Part print with two shaded views. Sizes in mm from the minimum x, y, z corner. Coordinates: 2 decimals unless noted, no trailing zeros. Write each loop counter-clockwise with the first axis right and the second up, starting at its lowest first coordinate (ties: lowest second). Pieces come first, ordered by that corner, then holes. Notation, with made-up numbers: M 80.25,19.5 L 101.25,19.5 A6 cw 101.25,23.5 Z; hole C 10,81.25 d7. An arc over 180 degrees is marked long. One line per question, with ' | ' between items. Start each with the question number.
(1) Cut at A-A (x = 18.5). Write the cut outline in (y, z), plus the area to 3 significant figures.
(2) Wall check: probe 1 along X at (y, z) = (2, 18.5); probe 2 along Z at (x, y) = (19, 1); probe 3 along Z at (x, y) = (13.5, 4). Give the ranges that are in metal, low to high.
(3) Cut at B-B (z = 18.5). Write the cut outline in (x, y), plus the area to 3 significant figures.
(4) Flat gauge pins, fed straight in: pin 1 Ø3 at (x, y) = (6, 5.5) entering from +Z; pin 2 Ø1.5 at (x, y) = (25.5, 1) entering from +Z; pin 3 Ø1.5 at (y, z) = (3, 29.5) entering from -X. Where does each tip first touch, or does it go through?
(5) Cut at C-C (y = 4). Write the cut outline in (x, z), plus the area to 3 significant figures.
(6) Two-plate mould, pull along Z, no slides. Class the marked faces 1, 2 and 3: +Z half, -Z half, draft (parallel to the pull), parting line (faces both ways), or undercut.
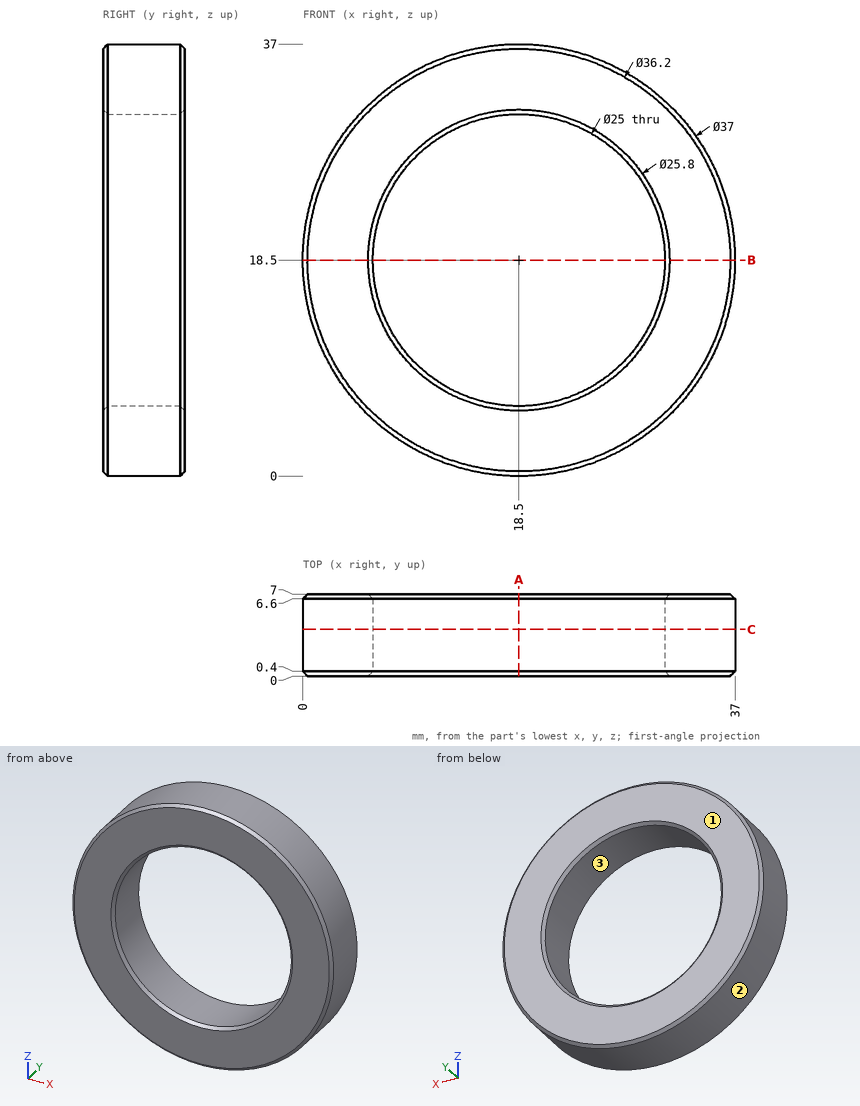
Filled in:
1) outline: M 0,0.4 L 0.4,0 L 6.6,0 L 7,0.4 L 7,5.6 L 6.6,6 L 0.4,6 L 0,5.6 Z; M 0,31.4 L 0.4,31 L 6.6,31 L 7,31.4 L 7,36.6 L 6.6,37 L 0.4,37 L 0,36.6 Z | area: 83.4 mm²
2) probe 1: 0 to 6, 31 to 37 | probe 2: 0.01 to 6.01, 30.99 to 36.99 | probe 3: 0.69 to 7.04, 29.96 to 36.31
3) outline: M 0,0.4 L 0.4,0 L 5.6,0 L 6,0.4 L 6,6.6 L 5.6,7 L 0.4,7 L 0,6.6 Z; M 31,0.4 L 31.4,0 L 36.6,0 L 37,0.4 L 37,6.6 L 36.6,7 L 31.4,7 L 31,6.6 Z | area: 83.4 mm²
4) pin 1: z = 33.37 | pin 2: z = 35.91 | pin 3: x = 3.1
5) outline: C 18.5,18.5 d37; hole C 18.5,18.5 d25 | area: 584 mm²
6) face 1: draft | face 2: parting line | face 3: undercut
